Design review of the part built by this model. Coordinates are the model's own, in mm. A direction names the side the tool comes from. Round coordinates to 2 decimals unless told otherwise and drop trailing zeros. Loops run counter-clockwise (first coordinate to the right, second up) from the corner with the lowest first, then second, coordinate; pieces in that order, holes last. Notation, with made-up numbers: M 70,34.25 L 85,34.25 A31 cw 85,72.25 Z; hole C -32,-10 d6. An arc over 180 degrees is marked long. One line per item, written item: value. Start each with the question number.
Item 1: Clearance check with a flat-ended pin moving along its axis: pin 1 (1 mm diameter, centred on x = -0.5, z = -1, fed in from -Y). State where the tip first meets the part, or that it passes through.
Item 2: Mouldability with a two-part tool opening along Z and no side actions: class faces 3 (the flat face through (0, 2.5, 0)), 4 (the flat face through (-2.838, 2.993, -7.726)), 5 (the flat face through (0, 3.5, 0)) as released by +Z, released by -Z, zero draft, split by the parting line, or undercut.
Item 3: We need section D-D (z = 11.5). Write out the cut boundary in (x, y).
Item 4: We need section C-C (x = 2.75). Write out the cut boundary in (y, z), then the cut area to 3 significant figures.
Item 5: For faces 1 (the flat face through (2, 0, -1)), 2 (the cylindrical face through (-3.233, 1.232, 1.341)), list the 3-axis set-ups (+Z, -Z, +X, -X, +Y, -Y) from which the entire face can be reached by the end or side of a thin tool; tool diameter is ignored.
Item 6: We need section A-A (z = -5.5). Write out the cut boundary in (x, y).
Item 7: For line 1 along Y through (x, z) = (-2.25, 6.5); line 2 along X through (y, z) = (3.2, -15.5); line 3 along X through (y, z) = (3, 9.5), list the stretches that pass through material, from the lowest coordinate up.
Item 8: We need section B-B (y = 0.3). Write out the cut boundary in (x, z).
Autodesk Inventor part; units mm, degrees
ref_plane "YZ Plane" through (0, 0, 0) normal (1, 0, 0) x (0, 1, 0)
ref_plane "XZ Plane" through (0, 0, 0) normal (0, 1, 0) x (-1, 0, 0)
ref_plane "XY Plane" through (0, 0, 0) normal (0, 0, 1) x (1, 0, 0)
sketch "Skizze1" plane through (0, 0, 0) normal (0, 1, 0) x (-1, 0, 0)
  circle A0 centre (0, 0) radius 1.75
  circle A1 centre (0, 0) radius 3.5
  dimension "d2" = 3.5
  dimension "d3" = 7
extrude "Extrusion1" add sketch "Skizze1" along normal blind 2.5
sketch "Skizze2" plane through (0, 2.5, 0) normal (0, 1, 0) x (1, 0, 0)
  line L0 (-2, 17.5) -> (2, 17.5)
  line L1 (2, 17.5) -> (2, -17.5)
  line L2 (2, -17.5) -> (-2, -17.5)
  line L3 (-2, -17.5) -> (-2, 17.5)
  line L4 (-2, 17.5) -> (2, -17.5) construction
  line L5 (2, 17.5) -> (-2, -17.5) construction
  circle A0 centre (0, 0) radius 3.5
  line L6 (3.5, 0) -> (2, -17.5)
  line L7 (-2, -17.5) -> (-3.5, 0)
  circle A1 centre (0, 0) radius 3.5
  line L8 (-3.5, 0) -> (-2, 17.5)
  line L9 (2, 17.5) -> (3.5, 0)
  dimension "d6" = 35
  dimension "d7" = 4
extrude "Extrusion2" add sketch "Skizze2" along normal blind 1 contours L0 L1 A0 L3 | L3 A0 L8 | L9 A0 L1 | A0 L1 L3 | L3 A0 L7 L8 | A0 L9 L6 L1 | A0 L1 L2 L3 | L3 L7 A0 | A0 L6 L1
sketch "Skizze3" plane through (0, 3.5, 0) normal (0, 1, 0) x (1, 0, 0)
  line L0 (-2, -17.5) -> (2, -17.5)
  point P0 (0, 0)
  point P1 (0, -15.5)
  point P2 (0, -13.5)
  point P3 (0, -11.5)
  point P4 (0, -9.5)
  point P5 (0, -7.5)
  point P6 (0, -5.5)
  point P7 (0, 5.5)
  point P8 (0, 7.5)
  point P9 (0, 9.5)
  point P10 (0, 11.5)
  point P11 (0, 13.5)
  point P12 (0, 15.5)
  dimension "d10" = 2
  dimension "d11" = 2
  dimension "d12" = 2
  dimension "d13" = 2
  dimension "d14" = 2
  dimension "d15" = 2
  dimension "d16" = 0
  dimension "d17" = 0
  dimension "d18" = 2
  dimension "d19" = 2
  dimension "d20" = 2
  dimension "d21" = 2
  dimension "d22" = 2
  dimension "d24" = 5.5
hole "Bohrung1" at (0, 3.5, 15.5) at (0, 3.5, 13.5) at (0, 3.5, 11.5) at (0, 3.5, 9.5) at (0, 3.5, 7.5) at (0, 3.5, 5.5) at (0, 3.5, -5.5) at (0, 3.5, -7.5) at (0, 3.5, -9.5) at (0, 3.5, -11.5) at (0, 3.5, -13.5) at (0, 3.5, -15.5) direction (0, -1, 0) diameter 1 depth 8 tip angle 118
fillet "Rundung1" radius 2 4 edges at (2, 3, 17.5) (-2, 3, 17.5) (2, 3, -17.5) (-2, 3, -17.5)
properties part number "horn"
A:
1. pin 1: y = 2.5
2. face 3: undercut
2. face 4: released by -Z
2. face 5: zero draft
3. outline: M -2.51,2.5 L -0.5,2.5 L -0.5,3.5 L -2.51,3.5 Z; M 0.5,2.5 L 2.51,2.5 L 2.51,3.5 L 0.5,3.5 Z
4. outline: M 0,-2.17 L 2.5,-2.17 L 2.5,-8.75 L 3.5,-8.75 L 3.5,8.75 L 2.5,8.75 L 2.5,2.17 L 0,2.17 Z
4. area: 28.3 mm2
5. face 1: +Z, -Z, +X, -X, -Y
5. face 2: -Y
6. outline: M -3.03,2.5 L -0.5,2.5 L -0.5,3.5 L -3.03,3.5 Z; M 0.5,2.5 L 3.03,2.5 L 3.03,3.5 L 0.5,3.5 Z
7. line 1: 2.5 to 3.5
7. line 2: -2.17 to -0.5, 0.5 to 2.17
7. line 3: -2.69 to -0.5, 0.5 to 2.69
8. outline: C 0,0 d7; hole C 0,0 d3.5
